from build123d import *

# Parameters (mm, degrees)
BOSS_EXTRUDE1_DEPTH     = 292.1
CUT_EXTRUDE1_DEPTH      = 305.17123736
CUT_EXTRUDE1_DEPTH_BACK = 305.17123736


with BuildPart() as part:
    # Sketch1 → Boss-Extrude1 (new body)
    with BuildSketch(Plane.XY):
        with BuildLine():
            Line((-2.54, 1.466469684), (-2.54, 7.520126744))
            ThreePointArc((-2.54, 7.520126744), (-6.874076643, 3.96875), (-7.7826208, -1.560358847))
            Line((-7.7826208, -1.560358847), (-2.54, 1.466469684))
        make_face()
        with BuildLine():
            ThreePointArc((-5.2426208, -5.959767898), (0, -7.9375), (5.2426208, -5.959767898))
            Line((5.2426208, -5.959767898), (0, -2.932939367))
            Line((0, -2.932939367), (-5.2426208, -5.959767898))
        make_face()
        with BuildLine():
            ThreePointArc((7.9375, 0), (6.448455484, 4.628318067), (2.54, 7.520126744))
            Line((2.54, 7.520126744), (2.54, 1.466469684))
            Line((2.54, 1.466469684), (7.7826208, -1.560358847))
            ThreePointArc((7.7826208, -1.560358847), (7.898685297, -0.784013281), (7.9375, 0))
        make_face()
        with BuildLine():
            Line((6.874076643, -3.96875), (0, 0))
            Line((0, 0), (-6.874076643, -3.96875))
            ThreePointArc((-6.874076643, -3.96875), (-6.139595043, -5.030832829), (-5.2426208, -5.959767898))
            Line((-5.2426208, -5.959767898), (0, -2.932939367))
            Line((0, -2.932939367), (5.2426208, -5.959767898))
            ThreePointArc((5.2426208, -5.959767898), (6.139595043, -5.030832829), (6.874076643, -3.96875))
        make_face()
        with BuildLine():
            Line((-6.874076643, -3.96875), (0, 0))
            Line((0, 0), (0, 7.9375))
            ThreePointArc((0, 7.9375), (-1.28703151, 7.832461691), (-2.54, 7.520126744))
            Line((-2.54, 7.520126744), (-2.54, 1.466469684))
            Line((-2.54, 1.466469684), (-7.7826208, -1.560358847))
            ThreePointArc((-7.7826208, -1.560358847), (-7.426626554, -2.801628862), (-6.874076643, -3.96875))
        make_face()
        with BuildLine():
            Line((0, 7.9375), (0, 0))
            Line((0, 0), (6.874076643, -3.96875))
            ThreePointArc((6.874076643, -3.96875), (7.426626554, -2.801628862), (7.7826208, -1.560358847))
            Line((7.7826208, -1.560358847), (2.54, 1.466469684))
            Line((2.54, 1.466469684), (2.54, 7.520126744))
            ThreePointArc((2.54, 7.520126744), (1.28703151, 7.832461691), (0, 7.9375))
        make_face()
        with BuildLine():
            Line((0, 63.5), (0, 7.9375))
            ThreePointArc((0, 7.9375), (1.28703151, 7.832461691), (2.54, 7.520126744))
            Line((2.54, 7.520126744), (2.54, 63.5))
            Line((2.54, 63.5), (0, 63.5))
        make_face()
        with BuildLine():
            ThreePointArc((-2.54, 7.520126744), (-1.28703151, 7.832461691), (0, 7.9375))
            Line((0, 7.9375), (0, 63.5))
            Line((0, 63.5), (-2.54, 63.5))
            Line((-2.54, 63.5), (-2.54, 7.520126744))
        make_face()
        with BuildLine():
            Line((-54.99261314, -31.75), (-6.874076643, -3.96875))
            ThreePointArc((-6.874076643, -3.96875), (-7.426626554, -2.801628862), (-7.7826208, -1.560358847))
            Line((-7.7826208, -1.560358847), (-56.26261314, -29.550295474))
            Line((-56.26261314, -29.550295474), (-54.99261314, -31.75))
        make_face()
        with BuildLine():
            ThreePointArc((-5.2426208, -5.959767898), (-6.139595043, -5.030832829), (-6.874076643, -3.96875))
            Line((-6.874076643, -3.96875), (-54.99261314, -31.75))
            Line((-54.99261314, -31.75), (-53.72261314, -33.949704526))
            Line((-53.72261314, -33.949704526), (-5.2426208, -5.959767898))
        make_face()
        with BuildLine():
            Line((54.99261314, -31.75), (6.874076643, -3.96875))
            ThreePointArc((6.874076643, -3.96875), (6.139595043, -5.030832829), (5.2426208, -5.959767898))
            Line((5.2426208, -5.959767898), (53.72261314, -33.949704526))
            Line((53.72261314, -33.949704526), (54.99261314, -31.75))
        make_face()
        with BuildLine():
            ThreePointArc((7.7826208, -1.560358847), (7.426626554, -2.801628862), (6.874076643, -3.96875))
            Line((6.874076643, -3.96875), (54.99261314, -31.75))
            Line((54.99261314, -31.75), (56.26261314, -29.550295474))
            Line((56.26261314, -29.550295474), (7.7826208, -1.560358847))
        make_face()
    extrude(amount=BOSS_EXTRUDE1_DEPTH)

    # Sketch2 → Cut-Extrude1 (cut, two sides: drawn at the far end of the back side and taken through both)
    with BuildSketch(Plane.XY.offset(292.1).offset(-CUT_EXTRUDE1_DEPTH_BACK)):
        with BuildLine():
            Line((0, 3.81), (3.81, 0))
            ThreePointArc((3.81, 0), (-2.694076836, -2.694076836), (0, 3.81))
        make_face()
    extrude(amount=CUT_EXTRUDE1_DEPTH + CUT_EXTRUDE1_DEPTH_BACK, mode=Mode.SUBTRACT)


solid = part.part
Design review of the part built by this model. Coordinates are the model's own, in mm. A direction names the side the tool comes from. Round coordinates to 2 decimals unless told otherwise and drop trailing zeros. Write each loop counter-clockwise with the first axis right and the second up, starting at its lowest first coordinate (ties: lowest second). Pieces come first, ordered by that corner, then holes. Notation, with made-up numbers: (8.5, -7.5) - (44.5, -7.5) arc R11 ccw to (44.5, -2.5) - close; hole circle Ø10 at (1, 69.5). An arc over 180 degrees is marked (long way). Return JSON: item names as keys, results as strings. Group by question number.
Item 1: The part is to be moulded in two halves that separate along Y. For faces 4 (the face through (-2.604, -2.781, 144.005)), 5 (the face through (-2.54, 36, 144)), 6 (the face through (-29.82, -20.15, 144.01)), say which applies: pulls with the +Y half, pulls with the -Y half, needs draft (parallel to the pull), parting line crosses it, or undercut.
Item 2: We need section C-C on x = 42. Write out the cut boundary in (y, z).
Item 3: Insertion check: P1, Ø6, axis at x = -15.5, z = 95, coming from the +Y side; P2, Ø1.5, axis at x = -41, z = 65.5, coming from the -Y side; P3, Ø12, axis at y = 36.5, z = 168, coming from the -X side. Each pin has a flat end and moves straight along its axis. Give the tip position at first contact, or say it passes through.
Item 4: For probe 1 along Y at (x, z) = (0, 117); probe 2 along X at (y, z) = (39, 113); probe 3 along Y at (x, z) = (-14.5, 260), list the stretches that pass through material, from the lowest coordinate up. Write a range as [from, to].
Item 5: We need section A-A on z = 220. Write out the cut boundary in (x, y) (1 decimal).
Item 6: We need section B-B on y = 48.5. Write out the cut boundary in (x, z).
Item 7: Machinability: for faces 1 (the face through (2.54, 35, 144)), 2 (the face through (29.143, -19.759, 144.005)), 3 (the face through (4, -3, 292.1)), which of the approach directions +Z, -Z, +X, -X, +Y, -Y give a long, thin tool a straight path to every point of the face, cutting with its end or side? Answer none if there is none.
Model answer:
{
 "1": {"face 4": "undercut", "face 5": "needs draft", "face 6": "pulls with the -Y half"},
 "2": {"outline": "(-27.18, 0) - (-21.32, 0) - (-21.32, 292.1) - (-27.18, 292.1) - close"},
 "3": {"P1": "stops at y = -4.28", "P2": "stops at y = -27.04", "P3": "stops at x = -2.54"},
 "4": {"probe 1": "y = [-7.94, -3.81], [3.81, 63.5]", "probe 2": "x = [-2.54, 2.54]", "probe 3": "y = [-11.3, -5.44]"},
 "5": {"outline": "(-56.3, -29.6) - (-53.7, -33.9) - (-5.2, -6) arc R7.9 ccw to (5.2, -6) - (53.7, -33.9) - (56.3, -29.6) - (7.8, -1.6) arc R7.9 ccw to (2.5, 7.5) - (2.5, 63.5) - (-2.5, 63.5) - (-2.5, 7.5) arc R7.9 ccw to (-7.8, -1.6) - close; hole (0, 3.8) arc R3.8 ccw (long way) to (3.8, 0) - close"},
 "6": {"outline": "(-2.54, 0) - (2.54, 0) - (2.54, 292.1) - (-2.54, 292.1) - close"},
 "7": {"face 1": "+Z, -Z, +X, +Y", "face 2": "+Z, -Z, -Y", "face 3": "+Z, +X, -X, +Y, -Y"}
}
